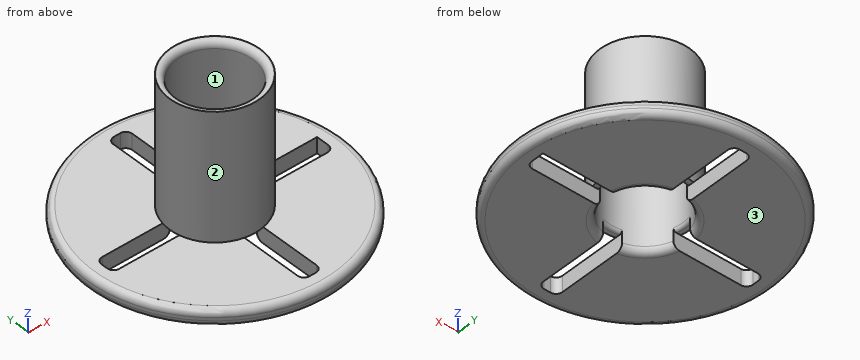
```python
from build123d import *

# Parameters (mm, degrees)
SKETCH_R        = 40
PAD_DEPTH       = 5
SKETCH001_R     = 14.25
PAD001_DEPTH    = 40
SKETCH002_R     = 12
POCKET_DEPTH    = 45.001
POCKET001_DEPTH = 5
FILLET_R        = 2
FILLET001_R     = 2
FILLET002_R     = 1
FILLET003_R     = 2
FILLET004_R     = 2


with BuildPart() as part:
    # Sketch → Pad (new body)
    with BuildSketch(Plane.XY):
        Circle(SKETCH_R)
    extrude(amount=PAD_DEPTH)

    # Sketch001 (on Face3 of Pad) → Pad001 (join)
    with BuildSketch(Plane.XY.offset(5)):
        Circle(SKETCH001_R)
    extrude(amount=PAD001_DEPTH)

    # Sketch002 (on Face5 of Pad001) → Pocket (cut, through all)
    with BuildSketch(Plane.XY.offset(45)):
        Circle(SKETCH002_R)
    extrude(amount=-POCKET_DEPTH, mode=Mode.SUBTRACT)

    # Sketch003 (on Face2 of Pocket) → Pocket001 (cut)
    with BuildSketch(Plane(origin=(0, 0, 0), x_dir=(1, 0, 0), z_dir=(0, 0, -1))):
        Polygon((-3, 35), (-3, 3), (-35, 3), (-35, -3), (-3, -3), (-3, -35), (3, -35), (3, -3), (35, -3), (35, 3), (3, 3), (3, 35), align=None)
    extrude(amount=-POCKET001_DEPTH, mode=Mode.SUBTRACT)

    # Fillet
    fillet_edges = [part.edges().sort_by_distance(p)[0] for p in [
        (-3, -35, 2.5),
        (3, -35, 2.5),
        (35, -3, 2.5),
        (-35, -3, 2.5),
        (-35, 3, 2.5),
        (-3, 35, 2.5),
        (3, 35, 2.5),
    ]]
    fillet(fillet_edges, radius=FILLET_R)

    # Fillet001
    fillet001_edges = [part.edges().sort_by_distance(p)[0] for p in [
        (8.485281, -8.485281, 0),
        (8.485281, 8.485281, 0),
        (-8.485281, 8.485281, 0),
        (-8.485281, -8.485281, 0),
    ]]
    fillet(fillet001_edges, radius=FILLET001_R)

    # Fillet002
    fillet002_edges = [part.edges().sort_by_distance(p)[0] for p in [
        (0, -12, 5),
        (11.904356, -1.512052, 5),
        (0, 12, 5),
        (-12, 0, 5),
    ]]
    fillet(fillet002_edges, radius=FILLET002_R)

    # Fillet003
    fillet003_edges = [part.edges().sort_by_distance(p)[0] for p in [
        (-40, 0, 5),
        (-40, 0, 0),
    ]]
    fillet(fillet003_edges, radius=FILLET003_R)

    # Fillet004
    fillet004_edges = [part.edges().sort_by_distance(p)[0] for p in [
        (-12, 0, 45),
    ]]
    fillet(fillet004_edges, radius=FILLET004_R)


solid = part.part
```
Design review of the part built by this model. Coordinates are the model's own, in mm. Face numbers are marked on the shaded views. Round coordinates to 2 decimals unless told otherwise and drop trailing zeros. Write each loop counter-clockwise with the first axis right and the second up, starting at its lowest first coordinate (ties: lowest second). Pieces come first, ordered by that corner, then holes. Notation, with made-up numbers: (67.5, 28) -> (94.5, 28) arc R21 cw to (94.5, 36) -> close; hole circle Ø3 at (55.5, 62.5). An arc over 180 degrees is marked (long way). Write item = value, one per line. Start each with the question number.
1) Wall thickness on probe 1 along Y at (x, z) = (0, 31); probe 2 along Z at (x, y) = (-35.5, -12): over which ranges is each line inside the solid? List them lowest first. Write a range as from..to.
2) Clearance check with flat-ended pins moving along their axes: pin 1 (6 mm diameter, centred on x = 11.5, z = 30, fed in from -Y); pin 2 (5 mm diameter, centred on x = -29, y = 28.5, fed in from -Z); pin 3 (1.8 mm diameter, centred on x = 27.5, z = 2.5, fed in from -Y); pin 4 (12 mm diameter, centred on x = -22, z = 35.5, fed in from +Y). State where each tip first meets the part, or that it passes through.
3) Take a section at C-C, the plane z = 30. State the section outline as (x, y) points, plus the area to 3 significant figures.
4) Take a section at A-A, the plane y = 0. State the section outline as (x, z) points, plus the area to 3 significant figures.
5) Mouldability with a two-part tool opening along Y and no side actions: class the marked faces 1, 2 and 3 as +Y half, -Y half, draft (parallel to the pull), parting line (faces both ways), or undercut.
Results list:
q1.probe_1 = -14.25..-12, 12..14.25
q1.probe_2 = 0..5
q2.pin_1 = -11.44
q2.pin_2 = 0.01
q2.pin_3 = -29.87
q2.pin_4 = through
q3.outline = circle Ø28.5 at (0, 0); hole circle Ø24 at (0, 0)
q3.area = 186 mm²
q4.outline = (-40, 2) arc R2 ccw to (-38, 0) -> (-35, 0) -> (-35, 5) -> (-38, 5) arc R2 ccw to (-40, 3) -> close; (-14.25, 5) -> (-13, 5) arc R1 ccw to (-12, 6) -> (-12, 43) arc R2 ccw to (-14, 45) -> (-14.25, 45) -> close; (12, 6) arc R1 ccw to (13, 5) -> (14.25, 5) -> (14.25, 45) -> (14, 45) arc R2 ccw to (12, 43) -> close; (35, 0) -> (38, 0) arc R2 ccw to (40, 2) -> (40, 3) arc R2 ccw to (38, 5) -> (35, 5) -> close
q4.area = 224 mm²
q5.face_1 = undercut
q5.face_2 = parting line
q5.face_3 = draft
